from build123d import *

# Parameters (mm, degrees)
F0_W     = 159.7669422626
F0_H     = 59.7716327757
F1_DEPTH = 25
F2_W     = 36.0885336995
F2_H     = 59.7716327757
F2_W_2   = 36.0885262489
F3_DEPTH = 60
F4_R     = 5


with BuildPart() as f1:
    # F0 (on Top) → F1 (new body)
    with BuildSketch(Plane.XY):
        with Locations((12.2174695134, 5.6388350204)):
            Rectangle(F0_W, F0_H)
    extrude(amount=F1_DEPTH)

    # F2 (on face) → F3 (join)
    with BuildSketch(Plane.XY.offset(25)):
        with Locations((-5.8267973363, 5.6388350204)):
            Rectangle(F2_W, F2_H)
        with Locations((30.2617326379, 5.6388350204)):
            Rectangle(F2_W_2, F2_H)
    extrude(amount=F3_DEPTH)

    # F4
    f4_edges = [f1.edges().sort_by_distance(p)[0] for p in [
        (-23.871064, -24.246981, 55),
        (-23.871064, 35.524651, 55),
        (48.305996, -24.246981, 55),
        (-45.768533, -24.246981, 25),
        (-45.768533, 35.524651, 25),
        (70.203468, -24.246981, 25),
        (70.203468, 35.524651, 25),
        (48.305996, 35.524651, 55),
        (-67.666002, 5.638835, 25),
        (92.100941, 5.638835, 25),
        (48.305996, 5.638835, 85),
        (-23.871064, 5.638835, 85),
        (12.217466, 35.524651, 85),
        (12.217466, -24.246981, 85),
    ]]
    fillet(f4_edges, radius=F4_R)


solid = f1.part
The listing builds one solid part. Answer for the finished solid, in the listing's coordinates (mm). A direction names the side the tool comes from. Coordinates: 2 decimals unless noted, no trailing zeros. Loops run counter-clockwise (first coordinate to the right, second up) from the corner with the lowest first, then second, coordinate; pieces in that order, holes last. Notation, with made-up numbers: (-21.75, -27) -> (5.25, -27) arc R14 ccw to (5.25, -7) -> close; hole circle Ø9 at (-2.75, 75). An arc over 180 degrees is marked (long way). Answer in a Markdown table with one row per item. Add a question column.
1. The part is cut by section B-B, the plane x = 69. Write down the section's boundary in (y, z).
2. Flat-ended cylindrical pins translate along their axes: P1, Ø19.5, axis at x = -52.5, y = -0.5, coming from the +Z side; P2, Ø15, axis at y = 16, z = 43, coming from the +X side. Find the tip coordinate at first contact, or state that the pin passes through.
3. The part is cut by section C-C, the plane y = 23. Write down the section's boundary in (x, z).
4. The part is cut by section A-A, the plane z = 35. Write down the section's boundary in (x, y), then the cut area to 3 significant figures.
5. Consider line 1 (X direction, y = -18, z = 80); line 2 (Z direction, x = -53.5, y = 18); line 3 (X direction, y = -12, z = 24). Determine where each line is inside the solid, lowest interval first. Write a range as [from, to].
6. For faces 1 (the cylindrical face through (68.045, 34.099, 23.496)), 2 (the cylindrical face through (-42.927, 34.099, 23.496)), 3 (the cylindrical face through (46.802, -22.821, 50.42)), 4 (the cylindrical face through (-22.37, -22.82, 50.42)), determine the directions among +Z, -Z, +X, -X, +Y, -Y from which every point of the face is accessible in a straight line to the end or side of a thin tool.
Answer below:
| question | item | result |
|---|---|---|
| 1 | outline | (-24.25, 0) -> (35.52, 0) -> (35.52, 20) arc R5 ccw to (30.52, 25) -> (-19.25, 25) arc R5 ccw to (-24.25, 20) -> close |
| 2 | P1 | z = 25 |
| 2 | P2 | x = 48.31 |
| 3 | outline | (-67.67, 0) -> (92.1, 0) -> (92.1, 20) arc R5 ccw to (87.1, 25) -> (48.31, 25) -> (48.31, 80) arc R5 ccw to (43.31, 85) -> (-18.87, 85) arc R5 ccw to (-23.87, 80) -> (-23.87, 25) -> (-62.67, 25) arc R5 ccw to (-67.67, 20) -> close |
| 4 | outline | (-23.87, -19.25) arc R5 ccw to (-18.87, -24.25) -> (43.31, -24.25) arc R5 ccw to (48.31, -19.25) -> (48.31, 30.52) arc R5 ccw to (43.31, 35.52) -> (-18.87, 35.52) arc R5 ccw to (-23.87, 30.52) -> close |
| 4 | area | 4,290 mm2 |
| 5 | line 1 | [-23.87, 48.31] |
| 5 | line 2 | [0, 25] |
| 5 | line 3 | [-65.67, 90.1] |
| 6 | face 1 | +Z, +X, +Y |
| 6 | face 2 | +Z, -X, +Y |
| 6 | face 3 | +Z, +X, -Y |
| 6 | face 4 | +Z, -X, -Y |
